from build123d import *

# Parameters (mm, degrees)
BOSS_EXTRUDE1_DEPTH = 0.4318
SKETCH5_R           = 0.2286
BOSS_EXTRUDE2_DEPTH = 13.335


with BuildPart() as part:
    # Sketch2 → Boss-Extrude1 (new body)
    with BuildSketch(Plane(origin=(0, 0, 0), x_dir=(1, 0, 0), z_dir=(0, 1, 0))):
        with BuildLine():
            Line((-0.4445, 4.61413914), (-0.4445, 5.24913914))
            Line((-0.4445, 5.24913914), (0.4445, 5.24913914))
            Line((0.4445, 5.24913914), (0.4445, 4.61413914))
            ThreePointArc((0.4445, 4.61413914), (0, -4.6355), (-0.4445, 4.61413914))
        make_face()
    extrude(amount=BOSS_EXTRUDE1_DEPTH)

    # Sketch4 → Revolve1 (revolve)
    with BuildSketch(Plane.XY, mode=Mode.PRIVATE) as revolve1_sk:
        with BuildLine():
            Line((4.064, 1.0033), (4.064, 8.382))
            Line((4.064, 8.382), (0, 8.382))
            Line((0, 8.382), (0, 0.4318))
            Line((0, 0.4318), (4.6355, 0.4318))
            ThreePointArc((4.6355, 0.4318), (4.468111525, 0.835911525), (4.064, 1.0033))
        make_face()
    revolve(revolve1_sk.sketch.rotate(Axis((0, 8.382, 0), (0, -1, 0)), 180), axis=Axis((0, 8.382, 0), (0, -1, 0)))

    # Sketch5 → Boss-Extrude2 (add)
    with BuildSketch(Plane.XZ):
        with Locations(Location((-1.8542, -1.8542, 0), (0, 0, 90))):
            Circle(SKETCH5_R)
        with Locations(Location((1.8542, -1.8542, 0), (0, 0, 90))):
            Circle(SKETCH5_R)
        with Locations(Location((1.8542, 1.8542, 0), (0, 0, 90))):
            Circle(SKETCH5_R)
        with Locations(Location((-1.8542, 1.8542, 0), (0, 0, 90))):
            Circle(SKETCH5_R)
    extrude(amount=BOSS_EXTRUDE2_DEPTH)


solid = part.part
Input: part model. Units: mm. Frame: model coordinates. A direction names the side the tool comes from. Round coordinates to 2 decimals unless told otherwise and drop trailing zeros. Write each loop counter-clockwise with the first axis right and the second up, starting at its lowest first coordinate (ties: lowest second). Pieces come first, ordered by that corner, then holes.
1) Contact query for flat-ended pins moving along their axis: P1, Ø1, axis at x = 1, y = -4, coming from the -Z side; P2, Ø3, axis at x = -3.5, y = -0.5, coming from the -Z side; P3, Ø3, axis at x = -0.5, z = -3.5, coming from the -Y side; P4, Ø3, axis at y = -4, z = -1, coming from the +X side. Output: stop coordinate, or through.
2) Cut plane C-C (y = 2.5). Return the cut outline in (x, z).
3) Ray query, L1, parallel to Y at x = 2.5, z = -0.25; L2, parallel to Z at x = -1.75, y = -11.5; L3, parallel to Z at x = -2, y = -9. Return the intervals inside material, ascending.
4) Reachability of faces 1 (the cylindrical face through (0.2, 0.21, 4.63)), 2 (the cylindrical face through (0.881, 4.744, 3.967)) from +Z, -Z, +X, -X, +Y, -Y: full face, straight path, thin tool, end or side. Return the list, or none.
5) Cut plane B-B (x = 0). Return the cut outline in (y, z), then the cut area to 3 significant figures.
6) Cut plane D-D (y = -3). Return the cut outline in (x, z).
7) Cut plane A-A (z = 0). Return the cut outline in (x, y), then the cut area to 3 significant figures.
Geometry says:
1. P1: passes through
1. P2: stops at z = -4.14
1. P3: stops at y = 0
1. P4: stops at x = 2.08
2. outline: circle Ø8.13 at (0, 0)
3. L1: y = 0 to 8.38
3. L2: z = -2.06 to -1.65, 1.65 to 2.06
3. L3: z = -2.03 to -1.68, 1.68 to 2.03
4. face 1: +Y, -Y
4. face 2: +Y
5. outline: (0, -5.25) - (0.43, -5.25) - (0.43, -4.64) arc R0.57 ccw to (1, -4.06) - (8.38, -4.06) - (8.38, 4.06) - (1, 4.06) arc R0.57 ccw to (0.43, 4.64) - (0, 4.64) - close
5. area: 69.4 mm2
6. outline: circle Ø0.46 at (-1.85, -1.85); circle Ø0.46 at (-1.85, 1.85); circle Ø0.46 at (1.85, -1.85); circle Ø0.46 at (1.85, 1.85)
7. outline: (-4.64, 0) - (4.64, 0) - (4.64, 0.43) arc R0.57 ccw to (4.06, 1) - (4.06, 8.38) - (-4.06, 8.38) - (-4.06, 1) arc R0.57 ccw to (-4.64, 0.43) - close
7. area: 69.1 mm2
